from build123d import *

# Parameters (mm, degrees)
BOSS_EXTRUDE1_DEPTH = 12
BOSS_EXTRUDE2_DEPTH = 10
SKETCH4_W           = 13.751659717
SKETCH4_H           = 46.366215506
CUT_EXTRUDE1_DEPTH  = 10
SKETCH5_W           = 8.283570047
SKETCH5_H           = 65.91855038
CUT_EXTRUDE2_DEPTH  = 12


with BuildPart() as part:
    # Sketch2 → Boss-Extrude1 (new body)
    with BuildSketch(Plane(origin=(0, 0, 24.631338753), x_dir=(-1, 0, 0), z_dir=(0, 0, -1))):
        with BuildLine():
            Line((1.823068058, 603), (1.823068058, 663))
            Line((1.823068058, 663), (-1.882857166, 663))
            Line((-1.882857166, 663), (-1.882857166, 603))
            ThreePointArc((-1.882857166, 603), (-0.029894554, 601.147037388), (1.823068058, 603))
        make_face()
    extrude(amount=-BOSS_EXTRUDE1_DEPTH)

    # Sketch3 → Boss-Extrude2 (add)
    with BuildSketch(Plane(origin=(0, 0, 24.631338753), x_dir=(-1, 0, 0), z_dir=(0, 0, -1))):
        with BuildLine():
            Line((1.264894076, 663), (-1.303734146, 663))
            add(Edge.make_bspline(
                [(-1.303734146, 663), (-1.370231135, 661.776635062), (-1.590250356, 657.449713113), (-1.807353062, 651.572171687), (-1.896585428, 645.372497792), (-1.86904968, 640.732879739), (-1.745534221, 636.874692995), (-1.562088565, 633.805492743), (-1.371788238, 631.514699269), (-1.110556109, 629.246267473), (-0.82006967, 627.376977333), (-0.524480825, 625.91989796), (-0.290142677, 624.999996337), (-0.11575841, 624.480032386), (-0.0414459, 624.290359908)],
                knots=[0.640306561, 0.640306561, 0.640306561, 0.640306561, 0.664641164, 0.726373771, 0.757240075, 0.788106379, 0.818972683, 0.834405835, 0.849838987, 0.865272139, 0.88070529, 0.888421866, 0.896138442, 0.901180622, 0.901180622, 0.901180622, 0.901180622], degree=3))
            add(Edge.make_bspline(
                [(-0.0414459, 624.290359908), (0.033082795, 624.479947544), (0.208059728, 624.999712352), (0.443446447, 625.919346223), (0.740696225, 627.376087666), (1.033313538, 629.245045426), (1.297131595, 631.513177934), (1.490043391, 633.803752969), (1.676987934, 636.872742091), (1.804901792, 640.730785516), (1.837726863, 645.370369162), (1.755562421, 651.570140757), (1.545143008, 657.448413886), (1.33002573, 661.776072077), (1.264894076, 663)],
                knots=[0.516530112, 0.516530112, 0.516530112, 0.516530112, 0.521572291, 0.529288867, 0.537005443, 0.552438595, 0.567871747, 0.583304899, 0.598738051, 0.629604354, 0.660470658, 0.691336962, 0.75306957, 0.777413882, 0.777413882, 0.777413882, 0.777413882], degree=3))
        make_face()
    extrude(amount=BOSS_EXTRUDE2_DEPTH)

    # Sketch4 → Cut-Extrude1 (cut)
    with BuildSketch(Plane(origin=(0, 0, 14.631338753), x_dir=(-1, 0, 0), z_dir=(0, 0, -1))):
        with Locations((-1.173878519, 643.806595501)):
            Rectangle(SKETCH4_W, SKETCH4_H)
        with BuildLine():
            Line((1.027790464, 662.75), (-1.066900471, 662.75))
            add(Edge.make_bspline(
                [(-1.066900471, 662.75), (-1.236503852, 659.603485126), (-1.378670819, 656.455796636), (-1.57969897, 650.156856184), (-1.640644161, 647.006539015), (-1.627793637, 642.280065577), (-1.605967013, 640.704411435), (-1.51576118, 637.5585905), (-1.447339544, 635.987803899), (-1.241955745, 632.852473359), (-1.105208785, 631.287909819), (-0.807374159, 628.949508907), (-0.693510346, 628.171370392), (-0.487056782, 627.00741033), (-0.412632368, 626.619934288), (-0.245133833, 625.846680816), (-0.152824444, 625.460833735), (-0.040997635, 625.076764299)],
                knots=[0, 0, 0, 0, 0.25, 0.25, 0.5, 0.5, 0.625, 0.625, 0.75, 0.75, 0.875, 0.875, 0.9375, 0.9375, 0.96875, 0.96875, 1, 1, 1, 1], degree=3))
            add(Edge.make_bspline(
                [(-0.040997635, 625.076764299), (0.070840901, 625.459248905), (0.163415052, 625.843948539), (0.33153675, 626.615305535), (0.406338832, 627.002048611), (0.614008944, 628.164202165), (0.728805435, 628.941690519), (1.029518166, 631.279177553), (1.168319449, 632.844593533), (1.37765883, 635.983274427), (1.448032565, 637.557347723), (1.541893042, 640.707003283), (1.565447656, 642.281912238), (1.583609245, 647.006821426), (1.526236009, 650.157618773), (1.332376457, 656.455957525), (1.193802364, 659.603511067), (1.027790464, 662.75)],
                knots=[0, 0, 0, 0, 0.03125, 0.03125, 0.0625, 0.0625, 0.125, 0.125, 0.25, 0.25, 0.375, 0.375, 0.5, 0.5, 0.75, 0.75, 1, 1, 1, 1], degree=3))
        make_face(mode=Mode.SUBTRACT)
    extrude(amount=-CUT_EXTRUDE1_DEPTH, mode=Mode.SUBTRACT)

    # Sketch5 → Cut-Extrude2 (cut)
    with BuildSketch(Plane.XY.offset(36.631338753)):
        with Locations((0.019038526, 632.037504846)):
            Rectangle(SKETCH5_W, SKETCH5_H)
        with BuildLine():
            Line((1.632857166, 603), (1.632857166, 662.75))
            Line((1.632857166, 662.75), (-1.573068058, 662.75))
            Line((-1.573068058, 662.75), (-1.573068058, 603))
            ThreePointArc((-1.573068058, 603), (0.029894554, 601.397037388), (1.632857166, 603))
        make_face(mode=Mode.SUBTRACT)
    extrude(amount=-CUT_EXTRUDE2_DEPTH, mode=Mode.SUBTRACT)


solid = part.part
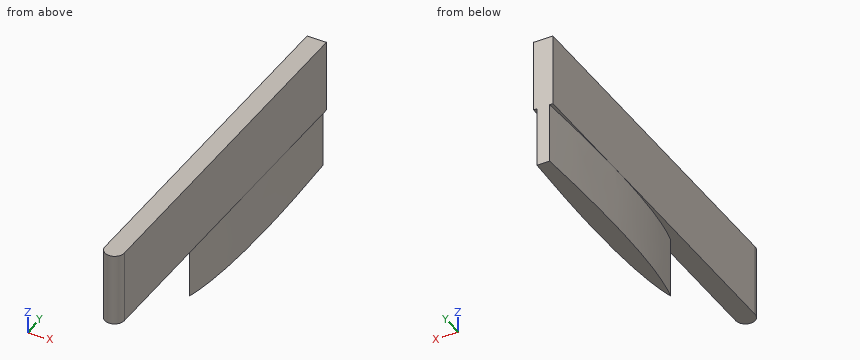
Geometry check sheet. Reference: the model listing, model coordinates, mm. Round coordinates to 2 decimals unless told otherwise and drop trailing zeros. Order: outer loops, then holes, each group sorted by start corner. A loop starts at its lowest first (then second) coordinate and runs counter-clockwise, first axis right, second up. Notation, with made-up numbers: (-23, 4) - (26, 4) arc R22 ccw to (26, 13) - close; hole circle Ø4 at (18, 58). An arc over 180 degrees is marked (long way). One line per question, with ' | ' between items. Start each with the question number.
(1) Thickness scan on L1, parallel to Z at x = -0.6, y = 627; L2, parallel to X at y = 645, z = 21.75; L3, parallel to Y at x = 1, z = 30.25. Record the ranges inside material, lowest first. Write a range as [from, to].
(2) Sectioned sample at A-A on y = 611. Record the cut outline in (x, z), and give its area (3 significant figures).
(3) Depth check by flat-ended pin: pin 1 Ø0.5 at (x, y) = (1.5, 658) entering from -Z; pin 2 Ø1.5 at (x, z) = (-1, 27.5) entering from -Y; pin 3 Ø1 at (x, y) = (-0.5, 617) entering from -Z. Enter the tip coordinate at first touch or a pass-through.
Conclusion:
1) L1: z = [24.63, 36.63] | L2: x = [-1.57, 1.63] | L3: y = [601.72, 662.75]
2) outline: (-1.57, 24.63) - (1.63, 24.63) - (1.63, 36.63) - (-1.57, 36.63) - close | area: 38.5 mm2
3) pin 1: stops at z = 14.63 | pin 2: stops at y = 601.42 | pin 3: stops at z = 24.63
